Design review of the part built by this model. Coordinates are the model's own, in mm. A direction names the side the tool comes from. Give positions to 0.01 mm unless a question says otherwise; leave off trailing zeros. Write each loop counter-clockwise with the first axis right and the second up, starting at its lowest first coordinate (ties: lowest second). Pieces come first, ordered by that corner, then holes.
```python
from build123d import *

# Parameters (mm, degrees)
CYLINDER060_R          = 3.5
CYLINDER060_DEPTH      = 10
CYLINDER060_ROLL_ANGLE = 90
CYLINDER059_R          = 1.8
CYLINDER059_DEPTH      = 48
CYLINDER059_ROLL_ANGLE = 90
CYLINDER058_R          = 3.5
CYLINDER058_DEPTH      = 10
CYLINDER058_ROLL_ANGLE = 90
CYLINDER057_R          = 3.5
CYLINDER057_DEPTH      = 10
CYLINDER057_ROLL_ANGLE = 90
CYLINDER051_R          = 1.8
CYLINDER051_DEPTH      = 100
CYLINDER051_ROLL_ANGLE = 90
CYLINDER056_R          = 2.2
CYLINDER056_DEPTH      = 100
CYLINDER056_ROLL_ANGLE = 90
CYLINDER053_R          = 21
CYLINDER053_DEPTH      = 8
CYLINDER053_ROLL_ANGLE = 90


with BuildPart() as cilindro060:
    # Cylinder060 → Cylinder060 (new body)
    with BuildSketch(Plane.XY):
        Circle(CYLINDER060_R)
    extrude(amount=CYLINDER060_DEPTH)


with BuildPart() as cilindro060_1:
    # Cylinder060 roll: moved
    add(cilindro060.part.rotate(Axis((0, 0, 0), (1, 0, 0)), CYLINDER060_ROLL_ANGLE))


with BuildPart() as cilindro060_2:
    # Cylinder060 placement: moved
    add(cilindro060_1.part.moved(Location((38, 41, -5.5))))


with BuildPart() as cilindro059:
    # Cylinder059 → Cylinder059 (new body)
    with BuildSketch(Plane.XY):
        Circle(CYLINDER059_R)
    extrude(amount=CYLINDER059_DEPTH)


with BuildPart() as cilindro059_1:
    # Cylinder059 roll: moved
    add(cilindro059.part.rotate(Axis((0, 0, 0), (1, 0, 0)), CYLINDER059_ROLL_ANGLE))


with BuildPart() as cilindro059_2:
    # Cylinder059 placement: moved
    add(cilindro059_1.part.moved(Location((38, 41, -5.5))))


with BuildPart() as cilindro058:
    # Cylinder058 → Cylinder058 (new body)
    with BuildSketch(Plane.XY):
        Circle(CYLINDER058_R)
    extrude(amount=CYLINDER058_DEPTH)


with BuildPart() as cilindro058_1:
    # Cylinder058 roll: moved
    add(cilindro058.part.rotate(Axis((0, 0, 0), (1, 0, 0)), CYLINDER058_ROLL_ANGLE))


with BuildPart() as cilindro058_2:
    # Cylinder058 placement: moved
    add(cilindro058_1.part.moved(Location((38, 41, 22.5))))


with BuildPart() as cilindro057:
    # Cylinder057 → Cylinder057 (new body)
    with BuildSketch(Plane.XY):
        Circle(CYLINDER057_R)
    extrude(amount=CYLINDER057_DEPTH)


with BuildPart() as cilindro057_1:
    # Cylinder057 roll: moved
    add(cilindro057.part.rotate(Axis((0, 0, 0), (1, 0, 0)), CYLINDER057_ROLL_ANGLE))


with BuildPart() as cilindro057_2:
    # Cylinder057 placement: moved
    add(cilindro057_1.part.moved(Location((38, 31, 8.5))))


with BuildPart() as cilindro051:
    # Cylinder051 → Cylinder051 (new body)
    with BuildSketch(Plane.XY):
        Circle(CYLINDER051_R)
    extrude(amount=CYLINDER051_DEPTH)


with BuildPart() as cilindro051_1:
    # Cylinder051 roll: moved
    add(cilindro051.part.rotate(Axis((0, 0, 0), (1, 0, 0)), CYLINDER051_ROLL_ANGLE))


with BuildPart() as cilindro051_2:
    # Cylinder051 placement: moved
    add(cilindro051_1.part.moved(Location((38, 80, 22.5))))


with BuildPart() as cilindro056:
    # Cylinder056 → Cylinder056 (new body)
    with BuildSketch(Plane.XY):
        Circle(CYLINDER056_R)
    extrude(amount=CYLINDER056_DEPTH)


with BuildPart() as cilindro056_1:
    # Cylinder056 roll: moved
    add(cilindro056.part.rotate(Axis((0, 0, 0), (1, 0, 0)), CYLINDER056_ROLL_ANGLE))


with BuildPart() as cilindro056_2:
    # Cylinder056 placement: moved
    add(cilindro056_1.part.moved(Location((38, 94, 8))))


with BuildPart() as cut045:
    # Cylinder053 → Cylinder053 (new body)
    with BuildSketch(Plane.XY):
        Circle(CYLINDER053_R)
    extrude(amount=CYLINDER053_DEPTH)


with BuildPart() as cut045_1:
    # Cylinder053 roll: moved
    add(cut045.part.rotate(Axis((0, 0, 0), (1, 0, 0)), CYLINDER053_ROLL_ANGLE))


with BuildPart() as cut045_2:
    # Cylinder053 placement: moved
    add(cut045_1.part.moved(Location((38, 35, 8.5))))

    # Cut040: cut Cilindro056
    add(cilindro056_2.part, mode=Mode.SUBTRACT)

    # Cut041: cut Cilindro051
    add(cilindro051_2.part, mode=Mode.SUBTRACT)

    # Cut042: cut Cilindro057
    add(cilindro057_2.part, mode=Mode.SUBTRACT)

    # Cut043: cut Cilindro058
    add(cilindro058_2.part, mode=Mode.SUBTRACT)

    # Cut044: cut Cilindro059
    add(cilindro059_2.part, mode=Mode.SUBTRACT)

    # Cut045: cut Cilindro060
    add(cilindro060_2.part, mode=Mode.SUBTRACT)


solid = cut045_2.part
```
(1) To check wall thickness, follow L1, parallel to Z at x = 38, y = 32.5; L2, parallel to Z at x = 37.5, y = 28.25; L3, parallel to X at y = 34, z = 6. State the ranges of each line that lie inside material, in increasing order.
Resolved:
L1: z = -12.5 to -9, -2 to 5.8, 10.2 to 19, 26 to 29.5
L2: z = -12.49 to -7.23, -3.77 to 5.04, 11.96 to 20.77, 24.23 to 29.49
L3: x = 17.15 to 37.08, 38.92 to 58.85
(2) Consider section C-C, the plane y = 33.25. Give the boundary of the cut face in (x, z), then the cut area to 3 significant figures.
Resolved:
outline: circle Ø42 at (38, 8.5); hole circle Ø7 at (38, -5.5); hole circle Ø7 at (38, 22.5); hole circle Ø4.4 at (38, 8)
area: 1,290 mm2
(3) Consider section A-A, the plane x = 38. Give the boundary of the cut face in (y, z).
Resolved:
outline: (27, -12.5) - (35, -12.5) - (35, -9) - (31, -9) - (31, -7.3) - (27, -7.3) - close; (27, -3.7) - (31, -3.7) - (31, -2) - (35, -2) - (35, 5.8) - (31, 5.8) - (31, 5) - (27, 5) - close; (27, 12) - (31, 12) - (31, 10.2) - (35, 10.2) - (35, 19) - (31, 19) - (31, 20.7) - (27, 20.7) - close; (27, 24.3) - (31, 24.3) - (31, 26) - (35, 26) - (35, 29.5) - (27, 29.5) - close
(4) Clearance check with flat-ended pins moving along their axes: P1, Ø3, axis at x = 38, z = -5.5, coming from the -Y side; P2, Ø11, axis at x = 38, z = -5.5, coming from the -Y side; P3, Ø6.5, axis at x = 38, z = 8.5, coming from the -Y side; P4, Ø2, axis at y = 30.5, z = 15.5, coming from the -X side. State where each tip first meets the part, or that it passes through.
Resolved:
P1: passes through
P2: stops at y = 27
P3: stops at y = 31
P4: stops at x = 17.88
(5) Consider section D-D, the plane z = 8.5. Give the boundary of the cut face in (x, y).
Resolved:
outline: (17, 27) - (34.5, 27) - (34.5, 31) - (35.86, 31) - (35.86, 35) - (17, 35) - close; (40.14, 31) - (41.5, 31) - (41.5, 27) - (59, 27) - (59, 35) - (40.14, 35) - close
(6) Tool access review of faces 1 (the face through (35.2, 29, 6.4)), 2 (the face through (35.42, 33.028, 24.865)), 3 (the face through (39.717, 29.028, 23.041)): name each direction out of +Z, -Z, +X, -X, +Y, -Y from which nothing blocks a thin tool from reaching the whole face with its end or side.
Resolved:
face 1: -Y
face 2: +Y
face 3: +Y, -Y
(7) Mouldability with a two-part tool opening along Z and no side actions: class faces 4 (the face through (57.4, 31.06, 0.46)), 5 (the face through (38, 35, 4)), 6 (the face through (35.2, 33, -7.6)) as pulls with the +Z half, pulls with the -Z half, needs draft (parallel to the pull), parting line crosses it, or undercut.
Resolved:
face 4: parting line crosses it
face 5: needs draft
face 6: undercut
(8) Consider section B-B, the plane z = 22.5. Give the boundary of the cut face in (x, y).
Resolved:
outline: (22.35, 27) - (36.2, 27) - (36.2, 31) - (34.5, 31) - (34.5, 35) - (22.35, 35) - close; (39.8, 27) - (53.65, 27) - (53.65, 35) - (41.5, 35) - (41.5, 31) - (39.8, 31) - close
